Geometry check sheet. Reference: the model listing, model coordinates, mm. A direction names the side the tool comes from. Round coordinates to 2 decimals unless told otherwise and drop trailing zeros. Order: outer loops, then holes, each group sorted by start corner. A loop starts at its lowest first (then second) coordinate and runs counter-clockwise, first axis right, second up. Notation, with made-up numbers: (70.5, 77.25) - (113.5, 77.25) arc R26 cw to (113.5, 113.25) - close; hole circle Ø8 at (24.5, 43.25). An arc over 180 degrees is marked (long way). Use a Markdown table: item, result. Add a question column.
(1) Access from +Z, -Z, +X, -X, +Y, -Y to the whole of each face (thin tool, end or side, straight path). Record for faces 5 (the face through (18, 19, 0)), 6 (the face through (15, 38, -5)).
(2) Section check C-C on x = 8.25. Record the boundary of the cut face in (y, z).
(3) Thickness scan on line 1 along Y through (x, z) = (15.75, 11.5); line 2 along Z through (x, y) = (5.5, 30); line 3 along Z through (x, y) = (1, 3.5). Record the ranges inside material, lowest first. Write a range as [from, to].
(4) Section check D-D on y = 23.5. Record the boundary of the cut face in (x, z), then the cut area to 3 significant figures.
(5) Section check A-A on x = 13. Record the boundary of the cut face in (y, z), then the cut area to 3 significant figures.
(6) Section check B-B on z = 0. Record the boundary of the cut face in (x, y).
(7) Mould release check, pull along Y, two halves, no side actions. Record for faces 1 (the face through (18, 35, -3)), 2 (the face through (20.495, 36.479, 0.451)), 3 (the face through (15, 0, -5)), 4 (the face through (18, 3, -3)): released by +Y, released by -Y, zero draft, split by the parting line, or undercut.
(8) Gauge pin test, flat ends, axial feed: P1, Ø5, axis at y = 23, z = -4, coming from the -X side; P2, Ø3, axis at x = 5, y = 9, coming from the -Z side; P3, Ø3, axis at y = 31, z = 2, coming from the -X side; P4, Ø3, axis at x = 9.5, z = -9.5, coming from the -Y side. Record the tip position at first contact, or that the pin passes through.
```python
from build123d import *

# Parameters (mm, degrees)
SKETCH1_R           = 18
SKETCH1_R_2         = 15
BOSS_EXTRUDE1_DEPTH = 35
SKETCH2_R           = 20.5
SKETCH2_R_2         = 15
BOSS_EXTRUDE2_DEPTH = 3
SKETCH3_R           = 20.5
SKETCH3_R_2         = 15
BOSS_EXTRUDE3_DEPTH = 3
SKETCH2_2_R         = 20.5
SKETCH2_2_R_2       = 15
BOSS_EXTRUDE4_DEPTH = 3


with BuildPart() as part:
    # Sketch1 → Boss-Extrude1 (new body)
    with BuildSketch(Plane(origin=(0, 0, 0), x_dir=(1, 0, 0), z_dir=(0, 1, 0))):
        with Locations(Location((0, 0, 0), (0, 0, 270))):
            Circle(SKETCH1_R)
        with Locations(Location((0, 0, 0), (0, 0, 270))):
            Circle(SKETCH1_R_2, mode=Mode.SUBTRACT)
    extrude(amount=BOSS_EXTRUDE1_DEPTH)

    # Sketch2 → Boss-Extrude2 (add)
    with BuildSketch(Plane(origin=(0, 0, 0), x_dir=(1, 0, 0), z_dir=(0, 1, 0))):
        with Locations(Location((0, 0, 0), (0, 0, 270))):
            Circle(SKETCH2_R)
        with Locations(Location((0, 0, 0), (0, 0, 270))):
            Circle(SKETCH2_R_2, mode=Mode.SUBTRACT)
    extrude(amount=BOSS_EXTRUDE2_DEPTH)

    # Sketch3 → Boss-Extrude3 (add)
    with BuildSketch(Plane(origin=(0, 35, 0), x_dir=(1, 0, 0), z_dir=(0, 1, 0))):
        with Locations(Location((0, 0, 0), (0, 0, 270))):
            Circle(SKETCH3_R)
        with Locations(Location((0, 0, 0), (0, 0, 270))):
            Circle(SKETCH3_R_2, mode=Mode.SUBTRACT)
    extrude(amount=BOSS_EXTRUDE3_DEPTH)

    # Sketch2_2 → Boss-Extrude4 (add)
    with BuildSketch(Plane(origin=(0, 0, 0), x_dir=(1, 0, 0), z_dir=(0, 1, 0))):
        with Locations(Location((0, 0, 0), (0, 0, 270))):
            Circle(SKETCH2_2_R)
        with Locations(Location((0, 0, 0), (0, 0, 270))):
            Circle(SKETCH2_2_R_2, mode=Mode.SUBTRACT)
    extrude(amount=BOSS_EXTRUDE4_DEPTH)

    # Split1
    split(bisect_by=Plane(origin=(0, 0, 0), x_dir=(0, 0, 1), z_dir=(1, 0, 0)), keep=Keep.TOP)


solid = part.part
```
Check sheet entries:
| question | item | result |
|---|---|---|
| 1 | face 5 | +X |
| 1 | face 6 | +Z, -Z, +X, -X, +Y |
| 2 | outline | (0, -18.77) - (3, -18.77) - (3, -16) - (35, -16) - (35, -18.77) - (38, -18.77) - (38, -12.53) - (0, -12.53) - close; (0, 12.53) - (38, 12.53) - (38, 18.77) - (35, 18.77) - (35, 16) - (3, 16) - (3, 18.77) - (0, 18.77) - close |
| 3 | line 1 | y = [0, 3], [35, 38] |
| 3 | line 2 | z = [-17.14, -13.96], [13.96, 17.14] |
| 3 | line 3 | z = [-17.97, -14.97], [14.97, 17.97] |
| 4 | outline | (0, -18) arc R18 ccw to (0, 18) - (0, 15) arc R15 cw to (0, -15) - close |
| 4 | area | 156 mm2 |
| 5 | outline | (0, -15.85) - (3, -15.85) - (3, -12.45) - (35, -12.45) - (35, -15.85) - (38, -15.85) - (38, -7.48) - (0, -7.48) - close; (0, 7.48) - (38, 7.48) - (38, 15.85) - (35, 15.85) - (35, 12.45) - (3, 12.45) - (3, 15.85) - (0, 15.85) - close |
| 5 | area | 418 mm2 |
| 6 | outline | (15, 0) - (20.5, 0) - (20.5, 3) - (18, 3) - (18, 35) - (20.5, 35) - (20.5, 38) - (15, 38) - close |
| 7 | face 1 | undercut |
| 7 | face 2 | zero draft |
| 7 | face 3 | released by -Y |
| 7 | face 4 | undercut |
| 8 | P1 | stops at x = 13.52 |
| 8 | P2 | stops at z = -17.66 |
| 8 | P3 | stops at x = 14.59 |
| 8 | P4 | passes through |
